Design review of the part built by this model. Coordinates are the model's own, in mm. A direction names the side the tool comes from. Give positions to 0.01 mm unless a question says otherwise; leave off trailing zeros. Write each loop counter-clockwise with the first axis right and the second up, starting at its lowest first coordinate (ties: lowest second). Pieces come first, ordered by that corner, then holes. Notation, with made-up numbers: M 29,81.25 L 57,81.25 A24 cw 57,117.25 Z; hole C 88,-14 d9. An arc over 180 degrees is marked long. Answer in a Markdown table with one row per item.
```python
from build123d import *

# Parameters (mm, degrees)
F1_DEPTH = 355.6


with BuildPart() as f1:
    # F0 (on Right) → F1 (new body)
    with BuildSketch(Plane.YZ):
        with BuildLine():
            Line((73.025, 76.2), (-73.025, 76.2))
            ThreePointArc((-73.025, 76.2), (-75.270064, 75.270064), (-76.2, 73.025))
            Line((-76.2, 73.025), (-76.2, -73.025))
            ThreePointArc((-76.2, -73.025), (-75.270064, -75.270064), (-73.025, -76.2))
            Line((-73.025, -76.2), (73.025, -76.2))
            ThreePointArc((73.025, -76.2), (75.270064, -75.270064), (76.2, -73.025))
            Line((76.2, -73.025), (76.2, 73.025))
            ThreePointArc((76.2, 73.025), (75.270064, 75.270064), (73.025, 76.2))
        make_face()
        with BuildLine():
            Line((-69.850001, -66.674999), (-69.850001, 66.675001))
            ThreePointArc((-69.850001, 66.675001), (-68.920065, 68.920065), (-66.675001, 69.850001))
            Line((-66.675001, 69.850001), (66.675001, 69.850001))
            ThreePointArc((66.675001, 69.850001), (68.920065, 68.920065), (69.850001, 66.675001))
            Line((69.850001, 66.675001), (69.850001, -66.674999))
            ThreePointArc((69.850001, -66.674999), (68.920065, -68.920063), (66.675001, -69.849999))
            Line((66.675001, -69.849999), (-66.675001, -69.849999))
            ThreePointArc((-66.675001, -69.849999), (-68.920065, -68.920063), (-69.850001, -66.674999))
        make_face(mode=Mode.SUBTRACT)
    extrude(amount=F1_DEPTH)


solid = f1.part
```
1) Add section A-A (y = -45). Write out the cut boundary in (x, z).
Geometry says:
| item | result |
|---|---|
| outline | M 0,-76.2 L 355.6,-76.2 L 355.6,-69.85 L 0,-69.85 Z; M 0,69.85 L 355.6,69.85 L 355.6,76.2 L 0,76.2 Z |
2) Add section C-C (x = 143). Write out the cut boundary in (y, z) (3 decimals), and give its area (3 significant figures).
Geometry says:
| item | result |
|---|---|
| outline | M -76.2,-73.025 A3.175 ccw -73.025,-76.2 L 73.025,-76.2 A3.175 ccw 76.2,-73.025 L 76.2,73.025 A3.175 ccw 73.025,76.2 L -73.025,76.2 A3.175 ccw -76.2,73.025 Z; hole M -69.85,-66.675 A3.175 ccw -66.675,-69.85 L 66.675,-69.85 A3.175 ccw 69.85,-66.675 L 69.85,66.675 A3.175 ccw 66.675,69.85 L -66.675,69.85 A3.175 ccw -69.85,66.675 Z |
| area | 3,710 mm^2 |
3) For faces 4 (the face through (175, 69.85, 1)), 5 (the face through (175, -1, -76.2)), list the 3-axis set-ups (+Z, -Z, +X, -X, +Y, -Y) from which the entire face can be reached by the end or side of a thin tool; tool diameter is ignored.
Geometry says:
| item | result |
|---|---|
| face 4 | +X, -X |
| face 5 | -Z, +X, -X, +Y, -Y |
4) To check wall thickness, follow probe 1 along Y at (x, z) = (166, -8.5); probe 2 along Z at (x, y) = (289, 69.5). State the ranges of each line that lie inside material, in increasing order. Write a range as [from, to].
Geometry says:
| item | result |
|---|---|
| probe 1 | [-76.2, -69.85], [69.85, 76.2] |
| probe 2 | [-76.2, -68.12], [68.12, 76.2] |
5) The part is to be moulded in two halves that separate along Y. For faces 1 (the face through (175, 76.2, -1)), 2 (the face through (0, -6, -73)), 3 (the face through (175, 1, -69.85)), say which applies: released by +Y, released by -Y, zero draft, split by the parting line, or undercut.
Geometry says:
| item | result |
|---|---|
| face 1 | released by +Y |
| face 2 | zero draft |
| face 3 | undercut |
